Autodesk Inventor part; units mm, degrees
ref_plane "YZ Plane" through (0, 0, 0) normal (1, 0, 0) x (0, 1, 0)
ref_plane "XZ Plane" through (0, 0, 0) normal (0, 1, 0) x (-1, 0, 0)
ref_plane "XY Plane" through (0, 0, 0) normal (0, 0, 1) x (1, 0, 0)
sketch "Sketch1" plane through (0, 0, 0) normal (1, 0, 0) x (0, 1, 0)
  line L0 (0, 0) -> (17, 0)
  line L1 (17, 0) -> (17, -2)
  line L2 (17, -2) -> (0, -2)
  line L3 (0, -2) -> (0, 0)
  line L4 (17, 0) -> (13, 6.9282)
  line L5 (17, 0) -> (25, 0) construction
  line L6 (13, 6.9282) -> (11.2679, 5.9282)
  line L7 (11.2679, 5.9282) -> (14.6906, 0)
  line L8 (0, 0) -> (-15, 25.9808)
  line L9 (0, 0) -> (30, 0) construction
  line L10 (-15, 25.9808) -> (-16.7321, 24.9808)
  line L11 (-16.7321, 24.9808) -> (-1.1547, -2)
  line L12 (-1.1547, -2) -> (0, -2)
  line L13 (-16.7321, 24.9808) -> (-16.7321, -2)
  line L14 (-15, 25.9808) -> (-15, -2)
  line L15 (-15, -2) -> (-16.7321, -2)
  line L16 (17, 0) -> (15.8453, -2)
  point P0 (-15, 21.9808)
  dimension "d0" = 17
  dimension "d1" = 2
  dimension "d2" = 8
  dimension "d3" = 120
  dimension "d4" = 2
  dimension "d5" = 30
  dimension "d6" = 120
  dimension "d7" = 2
extrude "Extrusion1" add sketch "Sketch1" along normal blind 98 contours L0 L16 L2 L3 | L3 L12 L11 L14 L8 | L7 L6 L4 L0 | L14 L11 L10 | L11 L14 L15 L13
sketch "Sketch2" plane through (98, 0, 0) normal (1, 0, 0) x (0, 0, -1)
  line L0 (-5.9282, 11.2679) -> (-5.9282, -3.4226)
  line L1 (0, 0) -> (-25.9808, -15)
  line L2 (-5.9282, -3.4226) -> (-2.9641, 12.9793)
  line L3 (-5.9282, 11.2679) -> (0, 14.6906)
  line L4 (-5.9282, -3.4226) -> (0, 0)
  line L5 (0, 0) -> (0, 14.6906)
  line L6 (-2.9641, 12.9793) -> (0, 14.6906)
extrude "Extrusion2" add sketch "Sketch2" against normal blind 2 contours L2 L3 L5 L1
sketch "Sketch3" plane through (0, 0, 0) normal (-1, 0, 0) x (0, 0, 1)
  line L0 (2.9641, 12.9793) -> (5.9282, -3.4226)
  line L1 (5.9282, -3.4226) -> (2.9641, 12.9793)
  line L2 (5.9282, 11.2679) -> (0, 14.6906)
  line L3 (2.9641, 12.9793) -> (0, 14.6906)
  line L4 (5.9282, -3.4226) -> (0, 0)
  line L5 (0, 14.6906) -> (0, 0)
  line L6 (0, 0) -> (5.9282, -3.4226)
extrude "Extrusion3" add sketch "Sketch3" against normal blind 2
properties part number "Name_card_case"
CAD build for the part. Positions are in the model's coordinates, mm. A direction names the side the tool comes from. Round coordinates to 2 decimals unless told otherwise and drop trailing zeros. Write each loop counter-clockwise with the first axis right and the second up, starting at its lowest first coordinate (ties: lowest second). Pieces come first, ordered by that corner, then holes.
(1) Slice it at B-B, the plane z = 13.25. Write the cut outline in (x, y), and give its area (3 significant figures).
(2) 3-axis set-ups, long thin cutter, end or side, ignore diameter. For faces 5 (the face through (48.314, 12.146, 6.435)), 6 (the face through (48.314, -7.395, 12.809)), 7 (the face through (48, 7, 0)): which of +Z, -Z, +X, -X, +Y, -Y reach the whole face in a straight line?
(3) Slice it at A-A, the plane x = 77.5. Write the cut outline in (y, z).
(4) Mould opens along Y. For faces 1 (the face through (97.014, 4.664, 4.467)), 2 (the face through (48, 7, -2)), 3 (the face through (48.31, -15.85, 25.49)), 4 (the face through (48, -15, 10)) say: pulls with the +Y half, pulls with the -Y half, needs draft (parallel to the pull), parting line crosses it, or undercut.
(5) Probe line 1 along Y through (x, z) = (63, 1.5); line 2 along Y through (x, z) = (23, 1); line 3 along X through (y, z) = (-0.5, 2.5). List the from-to ranges inside material, lowest first.
(6) Drop flat-ended pins along their axis: P1, Ø3, axis at x = 18, y = 2, coming from the +Z side; P2, Ø12, axis at x = 25, z = 11, coming from the +Y side; P3, Ø12, axis at x = 59, z = 7, coming from the +Y side. Give the stop position or say it passes through.
(7) Slice it at D-D, the plane z = 18.75. Write the cut outline in (x, y), and give its area (3 significant figures).
(8) Slice it at C-C, the plane y = 10. Write the cut outline in (x, z), and give its area (3 significant figures).
From the geometry:
1. outline: (0, -16.73) - (98, -16.73) - (98, -15) - (0, -15) - close; (0, -9.96) - (98, -9.96) - (98, -7.65) - (0, -7.65) - close
1. area: 396 mm2
2. face 5: +Z, +X, -X
2. face 6: +Z
2. face 7: none
3. outline: (-16.73, -2) - (-15, -2) - (-15, 21.98) - (-1.15, -2) - (15.85, -2) - (17, 0) - (13, 6.93) - (11.27, 5.93) - (14.69, 0) - (0, 0) - (-15, 25.98) - (-16.73, 24.98) - close
4. face 1: undercut
4. face 2: needs draft
4. face 3: pulls with the -Y half
4. face 4: undercut
5. line 1: y = -16.73 to -15, -3.18 to -0.87, 13.82 to 16.13
5. line 2: y = -16.73 to -15, -2.89 to -0.58, 14.11 to 16.42
5. line 3: x = 0 to 2, 96 to 98
6. P1: stops at z = 0
6. P2: stops at y = 14.11
6. P3: stops at y = 16.42
7. outline: (0, -16.73) - (98, -16.73) - (98, -15) - (0, -15) - close; (0, -13.13) - (98, -13.13) - (98, -10.83) - (0, -10.83) - close
7. area: 396 mm2
8. outline: (0, -2) - (98, -2) - (98, 3.5) - (96, 3.5) - (96, 0) - (2, 0) - (2, 3.5) - (0, 3.5) - close
8. area: 210 mm2
